For this review, use the dimensioned drawing (mm, ordinates from the lowest corner) and the shaded views. A direction names the side the tool comes from. Round coordinates to 2 decimals unless told otherwise and drop trailing zeros. Write each loop counter-clockwise with the first axis right and the second up, starting at its lowest first coordinate (ties: lowest second). Pieces come first, ordered by that corner, then holes.
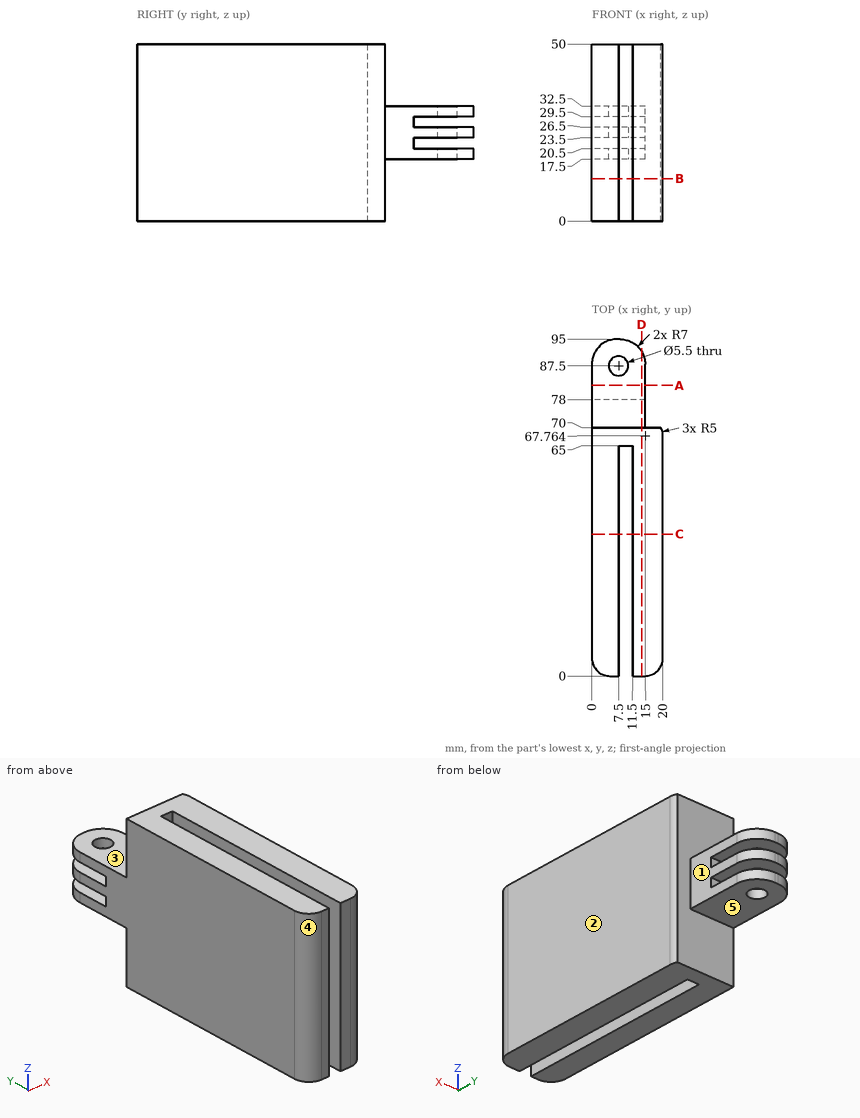
(1) We need section D-D, the plane x = 14. Give the boundary of the cut face in (y, z).
Geometry check:
outline: (0, 0) - (70, 0) - (70, 17.5) - (91.61, 17.5) - (91.61, 20.5) - (78, 20.5) - (78, 23.5) - (91.61, 23.5) - (91.61, 26.5) - (78, 26.5) - (78, 29.5) - (91.61, 29.5) - (91.61, 32.5) - (70, 32.5) - (70, 50) - (0, 50) - close
(2) We need section B-B, the plane z = 12. Give the boundary of the cut face in (x, y), and give its area (3 significant figures).
Geometry check:
outline: (0, 5) arc R5 ccw to (5, 0) - (7.5, 0) - (7.5, 65) - (11.5, 65) - (11.5, 0) - (15, 0) arc R5 ccw to (20, 5) - (20, 67.76) arc R5 ccw to (19.47, 70) - (0, 70) - close
area: 1,130 mm2
(3) We need section C-C, the plane y = 40. Give the boundary of the cut face in (x, z), and give its area (3 significant figures).
Geometry check:
outline: (0, 0) - (7.5, 0) - (7.5, 50) - (0, 50) - close; (11.5, 0) - (20, 0) - (20, 50) - (11.5, 50) - close
area: 800 mm2
(4) For pin 1 Ø1 at (x, z) = (16, 25) entering from -Y (3 decimals); pin 2 Ø1 at (x, y) = (9, 82.5) entering from -Z; pin 3 Ø5 at (x, z) = (4.5, 5.5) entering from +Y; pin 4 Ø1.5 at (x, y) = (18, 70) entering from -Z, all flat-tipped, find the tip position at first contact; note any pin that passes through.
Geometry check:
pin 1: stops at y = 0.025
pin 2: stops at z = 17.5
pin 3: stops at y = 70
pin 4: stops at z = 0
(5) We need section A-A, the plane y = 82. Give the boundary of the cut face in (x, z).
Geometry check:
outline: (0, 17.5) - (15, 17.5) - (15, 20.5) - (0, 20.5) - close; (0, 23.5) - (15, 23.5) - (15, 26.5) - (0, 26.5) - close; (0, 29.5) - (15, 29.5) - (15, 32.5) - (0, 32.5) - close
(6) For the marked faces 1, 2, 3, 4 and 5, list the 3-axis set-ups (+Z, -Z, +X, -X, +Y, -Y) from which the entire face can be reached by the end or side of a thin tool; tool diameter is ignored.
Geometry check:
face 1: +Z, -Z, +X, +Y
face 2: +Z, -Z, +X, +Y, -Y
face 3: +Z, +X, -X, +Y
face 4: +Z, -Z, -X, -Y
face 5: -Z, +X, -X, +Y
(7) For line 1 along X through (y, z) = (87.5, 31.7); line 2 along X through (y, z) = (57, 13); line 3 along Y through (x, z) = (12, 37), list the stretches that pass through material, from the lowest coordinate up.
Geometry check:
line 1: x = 0 to 4.75, 10.25 to 15
line 2: x = 0 to 7.5, 11.5 to 20
line 3: y = 0 to 70
